Design review of the part shown in the three views and the two pictorial views. Dimensions are in mm from the part's minimum x, y and z. A direction names the side the tool comes from. Give positions to 0.01 mm unless a question says otherwise; leave off trailing zeros. Loops run counter-clockwise (first coordinate to the right, second up) from the corner with the lowest first, then second, coordinate; pieces in that order, holes last.
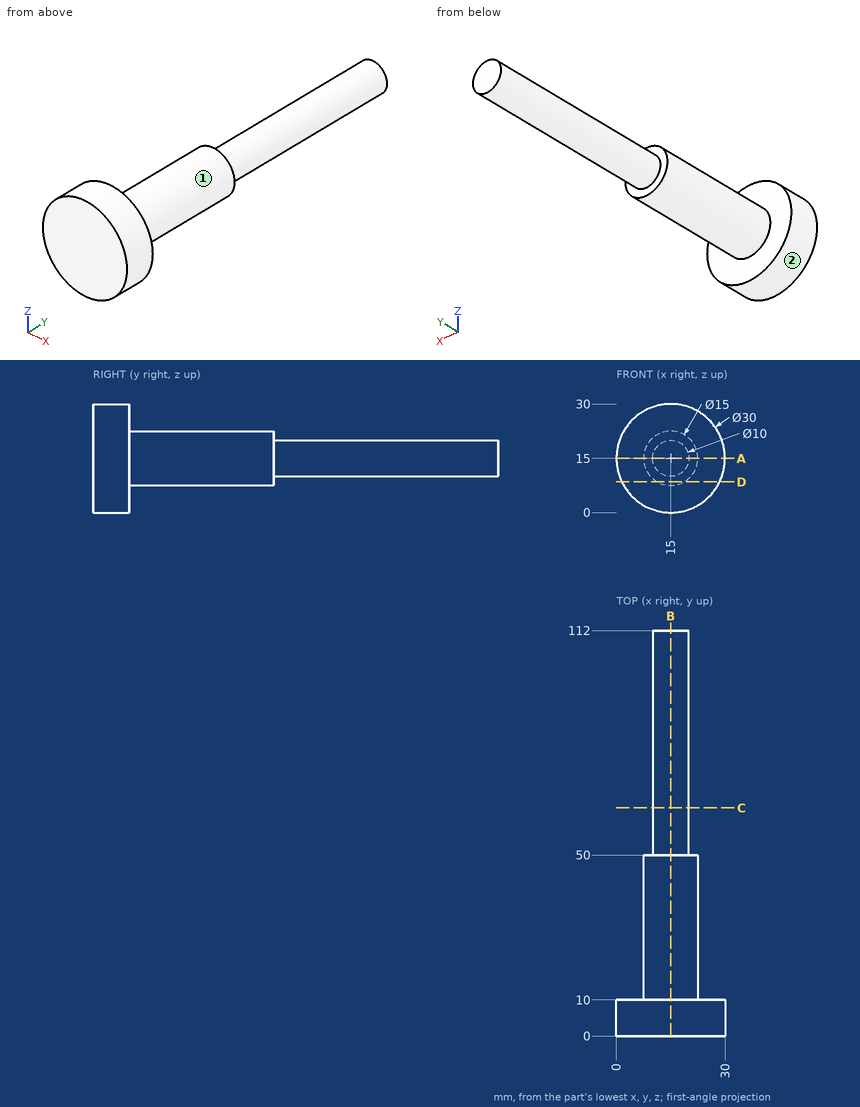
Q1. Machinability: for the marked faces 1 and 2, which of the approach directions +Z, -Z, +X, -X, +Y, -Y give a long, thin tool a straight path to every point of the face, cutting with its end or side? Answer none if there is none.
Answers:
face 1: +Y
face 2: +Y, -Y
Q2. For probe 1 along Y at (x, z) = (20.5, 13); probe 2 along Y at (x, z) = (23.75, 18.5); probe 3 along X at (y, z) = (29, 17.5), list the stretches that pass through material, from the lowest coordinate up.
Answers:
probe 1: y = 0 to 50
probe 2: y = 0 to 10
probe 3: x = 7.93 to 22.07
Q3. For pin 1 Ø10 at (x, y) = (10, 13) entering from +Z; pin 2 Ø10 at (y, z) = (22.5, 20.5) entering from -X; pin 3 Ø6 at (x, z) = (10.5, 24) entering from +Y; pin 4 Ø10 at (x, y) = (26.5, 70.5) entering from -Z, all flat-tipped, find the tip position at first contact; note any pin that passes through.
Answers:
pin 1: stops at z = 29.97
pin 2: stops at x = 7.52
pin 3: stops at y = 50
pin 4: passes through
Q4. Consider section B-B on x = 15. Give the boundary of the cut face in (y, z).
Answers:
outline: (0, 0) - (10, 0) - (10, 7.5) - (50, 7.5) - (50, 10) - (112, 10) - (112, 20) - (50, 20) - (50, 22.5) - (10, 22.5) - (10, 30) - (0, 30) - close
Q5. Consider section D-D on z = 8.5. Give the boundary of the cut face in (x, y).
Answers:
outline: (1.48, 0) - (28.52, 0) - (28.52, 10) - (18.74, 10) - (18.74, 50) - (11.26, 50) - (11.26, 10) - (1.48, 10) - close
Q6. Consider section A-A on z = 15. Give the boundary of the cut face in (x, y), plus the area to 3 significant figures.
Answers:
outline: (0, 0) - (30, 0) - (30, 10) - (22.5, 10) - (22.5, 50) - (20, 50) - (20, 112) - (10, 112) - (10, 50) - (7.5, 50) - (7.5, 10) - (0, 10) - close
area: 1,520 mm2
Q7. Consider section C-C on y = 63. Give the boundary of the cut face in (x, z).
Answers:
outline: circle Ø10 at (15, 15)
